```python
from build123d import *

# Parameters (mm, degrees)
F0_R      = 12.7
F1_DEPTH  = 187.325
F3_W      = 38.1
F3_H      = 25.4
F4_DEPTH  = 98.425
F5_W      = 38.1
F5_H      = 12.7
F8_D      = 12.7
F9_R      = 25.4
F10_DEPTH = 25.4
F11_W     = 125.786887
F11_H     = 48.075629
F12_DEPTH = 9.525


with BuildPart() as f1:
    # F0 (on Top) → F1 (new body, symmetric)
    with BuildSketch(Plane.XY):
        Circle(F0_R)
    extrude(amount=F1_DEPTH, both=True)

    # F3 (on offset) → F4 (join)
    with BuildSketch(Plane.XY.offset(187.325)):
        Rectangle(F3_W, F3_H)
    extrude(amount=F4_DEPTH)

    # F5 (on face) → F6 (revolve)
    with BuildSketch(Plane.XY.offset(285.75)):
        with Locations((0, 6.35)):
            Rectangle(F5_W, F5_H)
    revolve(axis=Axis((0, 0, 285.75), (1, 0, 0)))

    # F8 (through all)
    with Locations(Plane.YZ.offset(19.05)):
        with Locations((0, 285.75)):
            Hole(F8_D / 2)

    # F9 (on face) → F10 (join)
    with BuildSketch(Plane(origin=(0, 0, -187.325), x_dir=(1, 0, 0), z_dir=(0, 0, -1))):
        Circle(F9_R)
    extrude(amount=F10_DEPTH)

    # F11 (on Right) → F12 (cut, symmetric)
    with BuildSketch(Plane.YZ):
        with Locations((7.106817, 281.212815)):
            Rectangle(F11_W, F11_H)
    extrude(amount=F12_DEPTH, both=True, mode=Mode.SUBTRACT)


solid = f1.part
```
Read the model definition and answer for the solid it produces. Units are mm, in the model's axes. A direction names the side the tool comes from. Give positions to 0.01 mm unless a question says otherwise; leave off trailing zeros. Write each loop counter-clockwise with the first axis right and the second up, starting at its lowest first coordinate (ties: lowest second). Pieces come first, ordered by that corner, then holes. Notation, with made-up numbers: M -2,62.25 L 26,62.25 A30 cw 26,85.25 Z; hole C 79,83 d1. An arc over 180 degrees is marked long. Put each result on its own line as item: value. Start each with the question number.
1. The part is cut by section C-C, the plane y = 19.5. Give the vertices of the cut face in (x, z) (3 decimals).
2. Consider line 1 along Z through (x, y) = (-16.75, 0) (3 decimals); line 2 along Z through (x, y) = (-12, 0) (3 decimals); line 3 along Y through (x, z) = (12, 285). Determine where each line is inside the solid, lowest interval first.
3. The part is cut by section A-A, the plane y = 0. Give the vertices of the cut face in (x, z) (3 decimals), and give its area (3 significant figures).
4. The part is cut by section B-B, the plane z = 60. Give the vertices of the cut face in (x, y), and give its area (3 significant figures).
5. For a pull along Y with two mould halves and no side action, classify faces 1 (the flat face through (0, -12.7, 225)), 2 (the cylindrical face through (-14.354, 0.827, 292.046)), 3 (the flat face through (0, 0, -212.725)), 4 (the cylindrical face through (14.221, 0.827, 292.046)) as released by +Y, released by -Y, zero draft, split by the parting line, or undercut.
6. Which of the six approach directions +Z, -Z, +X, -X, +Y, -Y give full straight-line access (tool end or side, diameter ignored) to faces 5 (the cylindrical face through (-2.75, -12.4, 2.62)), 6 (the flat face through (14, 0, 187.325)), 7 (the flat face through (9.525, 0, 274))?
7. Each of these flat-tipped pins is pushed along its axis until it touches: pin 1 Ø9.5 at (x, y) = (-1, 2.5) entering from +Z (3 decimals); pin 2 Ø2 at (y, z) = (-12, -6.5) entering from +X; pin 3 Ø10 at (y, z) = (0, 285.75) entering from -X; pin 4 Ø10 at (y, z) = (5, 104) entering from +X. Where does it stop, or does it pass through?
Final values:
1. outline: M -16.276,-212.725 L 16.276,-212.725 L 16.276,-187.325 L -16.276,-187.325 Z
2. line 1: z = -212.725 to -187.325, 187.325 to 279.4, 292.1 to 298.45
2. line 2: z = -212.725 to 279.4, 292.1 to 298.45
2. line 3: y = -12.7 to -6.31, 6.31 to 12.7
3. outline: M -25.4,-212.725 L 25.4,-212.725 L 25.4,-187.325 L 12.7,-187.325 L 12.7,187.325 L 19.05,187.325 L 19.05,279.4 L 9.525,279.4 L 9.525,257.175 L -9.525,257.175 L -9.525,279.4 L -19.05,279.4 L -19.05,187.325 L -12.7,187.325 L -12.7,-187.325 L -25.4,-187.325 Z; M -19.05,292.1 L -9.525,292.1 L -9.525,298.45 L -19.05,298.45 Z; M 9.525,292.1 L 19.05,292.1 L 19.05,298.45 L 9.525,298.45 Z
3. area: 14,000 mm²
4. outline: C 0,0 d25.4
4. area: 507 mm²
5. face 1: released by -Y
5. face 2: undercut
5. face 3: zero draft
5. face 4: undercut
6. face 5: none
6. face 6: +X
6. face 7: +Z, +Y, -Y
7. pin 1: stops at z = 257.175
7. pin 2: stops at x = 6.35
7. pin 3: passes through
7. pin 4: stops at x = 12.7
